```python
from build123d import *

# Parameters (mm, degrees)
BOSS_EXTRUDE1_DEPTH = 882


with BuildPart() as part:
    # Sketch1 → Boss-Extrude1 (new body)
    with BuildSketch(Plane.XY):
        Polygon((-66.385092096, 0.943335029), (-16.885092096, 0.943335029), (0, 17.828427125), (16.590763052, 1.237664072), (66.090763052, 1.237664072), (66.090763052, 2.937664072), (66.090763052, 4.937664072), (79.090763052, 4.937664072), (79.090763052, 2.756664971), (68.385092096, 2.756664971), (68.385092096, -0.943335029), (16.885092096, -0.943335029), (0, -17.828427125), (-16.885092096, -0.943335029), (-66.385092096, -0.943335029), (-66.385092096, -2.043335029), (-66.385092096, -4.043335029), (-68.385092096, -4.043335029), (-80.385092096, -4.043335029), (-80.385092096, -2.043335029), (-68.385092096, -2.043335029), (-68.385092096, 0.943335029), align=None)
        Polygon((-15, 0), (0, 15), (15, 0), (0, -15), align=None, mode=Mode.SUBTRACT)
    extrude(amount=BOSS_EXTRUDE1_DEPTH)


solid = part.part
```
Read the model definition and answer for the solid it produces. Units are mm, in the model's axes. A direction names the side the tool comes from. Give positions to 0.01 mm unless a question says otherwise; leave off trailing zeros. Loops run counter-clockwise (first coordinate to the right, second up) from the corner with the lowest first, then second, coordinate; pieces in that order, holes last.
Item 1: The part is cut by section B-B (x = -31.5). Write down the section's boundary in (y, z), and give its area (3 significant figures).
Item 2: Find the intervals of material crossed by line 1 along X through (y, z) = (2.5, 535); line 2 along X through (y, z) = (2, 720); line 3 along Y through (x, z) = (71, 367), in increasing order.
Item 3: Each of these flat-tipped pins is pushed along its axis until it touches: pin 1 Ø1.5 at (y, z) = (-0.5, 473) entering from -X; pin 2 Ø13 at (x, z) = (-76.5, 617.5) entering from +Y; pin 3 Ø10 at (x, z) = (-13, 418.5) entering from +Y. Where does it stop, or does it pass through?
Item 4: The mould has two halves that part along Y. Classify faces 6 (the flat face through (-41, -0.943, 435)), 7 (the flat face through (41, 1.238, 435)), 8 (the flat face through (-7, -8, 435)): released by +Y, released by -Y, zero draft, split by the parting line, or undercut.
Item 5: For faces 1 (the flat face through (-42, 0.943, 435)), 2 (the flat face through (43, -0.943, 435)), 3 (the flat face through (8.18, 9.65, 434.83)), 4 (the flat face through (-73, -4.043, 435)), 5 (the flat face through (7, 8, 435)), determine the directions among +Z, -Z, +X, -X, +Y, -Y from which every point of the face is accessible in a straight line to the end or side of a thin tool.
Item 6: The part is cut by section A-A (z = 190). Write down the section's boundary in (x, y), and give its area (3 significant figures).
Item 7: The part is cut by section C-C (x = 38.5). Write down the section's boundary in (y, z).
Taken from the geometry:
1. outline: (-0.94, 0) - (0.94, 0) - (0.94, 882) - (-0.94, 882) - close
1. area: 1,660 mm2
2. line 1: x = -15.33 to -12.5, 12.5 to 15.33, 66.09 to 68.39
2. line 2: x = -15.83 to -13, 13 to 15.83, 66.09 to 68.39
2. line 3: y = 2.76 to 4.94
3. pin 1: stops at x = -68.39
3. pin 2: stops at y = -2.04
3. pin 3: stops at y = 9.83
4. face 6: released by -Y
4. face 7: released by +Y
4. face 8: undercut
5. face 1: +Z, -Z, -X, +Y
5. face 2: +Z, -Z, +X, -Y
5. face 3: +Z, -Z, +Y
5. face 4: +Z, -Z, -X, -Y
5. face 5: +Z, -Z
6. outline: (-80.39, -4.04) - (-66.39, -4.04) - (-66.39, -0.94) - (-16.89, -0.94) - (0, -17.83) - (16.89, -0.94) - (68.39, -0.94) - (68.39, 2.76) - (79.09, 2.76) - (79.09, 4.94) - (66.09, 4.94) - (66.09, 1.24) - (16.59, 1.24) - (0, 17.83) - (-16.89, 0.94) - (-68.39, 0.94) - (-68.39, -2.04) - (-80.39, -2.04) - close; hole (-15, 0) - (0, -15) - (15, 0) - (0, 15) - close
6. area: 455 mm2
7. outline: (-0.94, 0) - (1.24, 0) - (1.24, 882) - (-0.94, 882) - close
